Autodesk Inventor part; units mm, degrees
ref_plane "YZ Plane" through (0, 0, 0) normal (1, 0, 0) x (0, 1, 0)
ref_plane "XZ Plane" through (0, 0, 0) normal (0, 1, 0) x (-1, 0, 0)
ref_plane "XY Plane" through (0, 0, 0) normal (0, 0, 1) x (1, 0, 0)
sketch "Esquisse1" plane through (0, 0, 0) normal (1, 0, 0) x (0, 1, 0)
  line L0 (-30, 330) -> (30, 330)
  line L1 (30, 330) -> (30, -330)
  line L2 (30, -330) -> (-30, -330)
  line L3 (-30, -330) -> (-30, 330)
  line L4 (-30, 330) -> (30, -330) construction
  line L5 (30, 330) -> (-30, -330) construction
  point P0 (0, 0)
  dimension "d0" = 660
  dimension "d1" = 60
extrude "Extrusion1" add sketch "Esquisse1" along normal blind 18.55
sketch "Esquisse2" plane through (18.55, 0, 0) normal (1, 0, 0) x (0, 0, -1)
  circle A0 centre (-300, 0) radius 15
  circle A1 centre (0, 0) radius 15
  circle A2 centre (300, 0) radius 15
  line L0 (330, -30) -> (330, 30)
  line L1 (-330, 30) -> (-330, -30)
  line L2 (-330, 0) -> (330, 0) construction
  dimension "d4" = 30
  dimension "d5" = 30
  dimension "d6" = 30
extrude "Extrusion2" cut sketch "Esquisse2" against normal blind 18.55
fillet "Congé1" radius 30 1 edges at (9.275, 30, 330)
fillet "Congé2" radius 30 3 edges at (9.275, -30, 330) (9.275, 30, -330) (9.275, -30, -330)
properties part number "foot"
Here's how the part is built. I have some questions about the finished solid (model axes, mm). Give positions to 0.01 mm unless a question says otherwise; leave off trailing zeros. Order: outer loops, then holes, each group sorted by start corner. A loop starts at its lowest first (then second) coordinate and runs counter-clockwise, first axis right, second up. Notation, with made-up numbers: M 48.5,11.5 L 69.5,11.5 A15 cw 69.5,40.5 Z; hole C -10,-12 d9. An arc over 180 degrees is marked long. Use a Markdown table: item, result. Add a question column.
1. Suppose I cut it at B-B (x = 15.5). Give the number of separate pieces and of enclosed holes in the cut face, and give its area (3 significant figures).
2. Suppose I cut it at A-A (z = -5). List the corners of the cut face in (x, y) for me, and give its area (3 significant figures).
3. For pin 1 Ø3 at (x, y) = (11.5, 2.5) entering from +Z; pin 2 Ø4 at (x, y) = (11, 11.5) entering from +Z; pin 3 Ø4 at (x, y) = (2.5, -21) entering from +Z, each with a flat end and sliding along its axis, tell me the tip position at first contact or that it passes through.
4. If we mould it in two halves opening along Z, with no side actions, what happens to faces 1 (the cylindrical face through (9.405, -21.445, -320.979)), 2 (the cylindrical face through (9.405, -5.745, -313.856)), 3 (the flat face through (9, -30, -4))? For each: +Z half, -Z half, draft (parallel to the pull), parting line (faces both ways), or undercut.
5. I need wall thicknesses on probe 1 along Y at (x, z) = (11, 300); probe 2 along Z at (x, y) = (6.75, 5); probe 3 along Z at (x, y) = (10.5, -10). Which ranges of each line are inside material? Lowest first, please. Write a range as from..to.
Results list:
| question | item | result |
|---|---|---|
| 1 | separate pieces | 1 |
| 1 | enclosed holes | 3 |
| 1 | area | 36,700 mm² |
| 2 | outline | M 0,-30 L 18.55,-30 L 18.55,-14.14 L 0,-14.14 Z; M 0,14.14 L 18.55,14.14 L 18.55,30 L 0,30 Z |
| 2 | area | 588 mm² |
| 3 | pin 1 | stops at z = 329.98 |
| 3 | pin 2 | stops at z = 328.46 |
| 3 | pin 3 | stops at z = 323.22 |
| 4 | face 1 | -Z half |
| 4 | face 2 | undercut |
| 4 | face 3 | draft |
| 5 | probe 1 | y = -30..-15, 15..30 |
| 5 | probe 2 | z = -329.58..-314.14, -285.86..-14.14, 14.14..285.86, 314.14..329.58 |
| 5 | probe 3 | z = -328.28..-311.18, -288.82..-11.18, 11.18..288.82, 311.18..328.28 |
